The listing builds one solid part. Answer for the finished solid, in the listing's coordinates (mm). A direction names the side the tool comes from. Round coordinates to 2 decimals unless told otherwise and drop trailing zeros. Write each loop counter-clockwise with the first axis right and the second up, starting at its lowest first coordinate (ties: lowest second). Pieces come first, ordered by that corner, then holes. Notation, with made-up numbers: M -33,79 L -27,79 A21 cw -27,88 Z; hole C -21,28.5 d3. An arc over 180 degrees is marked long. One line per item, written item: value. Start each with the question number.
(1) For faces 1 (the cylindrical face through (-2.14, 9.52, 3.22)), 2 (the cylindrical face through (-17.19, 29.6, 3.22)), 3 (the cylindrical face through (-20.1, 40.8, 3.2)), determine the directions among +Z, -Z, +X, -X, +Y, -Y from which every point of the face is accessible in a straight line to the end or side of a thin tool.
(2) Consider probe 1 along Y at (x, z) = (-15.5, 4.75); probe 2 along Y at (x, z) = (-22, 2.5); probe 3 along Y at (x, z) = (-4, 4.75). Determine where each line is inside the solid, lowest interval first.
(3) Section C-C (y = 14.5) is taken. Determine the outline of the cut face in (x, z), plus the area to 3 significant figures.
(4) For a pull along Y with two mould halves and no side action, classify faces 4 (the cylindrical face through (-31.1, 39.5, 3.2)), 5 (the cylindrical face through (-24.469, 0.455, 3.219)), 6 (the cylindrical face through (-13.3, 72.9, 3.2)) as released by +Y, released by -Y, zero draft, split by the parting line, or undercut.
(5) Given P1, Ø10, axis at x = -32.5, y = 11, coming from the -Z side; P2, Ø1.9, axis at y = 22, z = 3, coming from the +X side, each flat-ended and moving along its own axis, determine where each tip first touches the part or whether it passes through.
(6) Section A-A (z = 3.5) is taken. Determine the outline of the cut face in (x, y), plus the area to 3 significant figures.
(7) Section B-B (x = -7) is taken. Determine the outline of the cut face in (y, z), plus the area to 3 significant figures.
(8) Section D-D (x = -16.5) is taken. Determine the outline of the cut face in (y, z).
```python
from build123d import *

# Parameters (mm, degrees)
F1_DEPTH = 6.35
F2_R     = 2


with BuildPart() as f1:
    # F0 (on Top) → F1 (new body)
    with BuildSketch(Plane.XY):
        Polygon((-24.87639, 0), (0, 0), (-1.76327, 10), (-17.76327, 10), (-17.76327, 30.2), (-5.325075, 30.2), (-12.9424, 73.4), (-37.289809, 73.4), (-35.52654, 63.4), (-19.52654, 63.4), (-19.52654, 40.2), (-31.964735, 40.2), align=None)
    extrude(amount=F1_DEPTH)

    # F2
    f2_edges = [f1.edges().sort_by_distance(p)[0] for p in [
        (-37.289809, 73.4, 3.175),
        (-35.52654, 63.4, 3.175),
        (-19.52654, 63.4, 3.175),
        (-31.964735, 40.2, 3.175),
        (-19.52654, 40.2, 3.175),
        (-12.9424, 73.4, 3.175),
        (-5.325075, 30.2, 3.175),
        (-17.76327, 30.2, 3.175),
        (-17.76327, 10, 3.175),
        (-1.76327, 10, 3.175),
        (0, 0, 3.175),
        (-24.87639, 0, 3.175),
    ]]
    fillet(f2_edges, radius=F2_R)


solid = f1.part
```
Recorded:
1. face 1: +Z, -Z, +X, +Y
1. face 2: +Z, -Z, +X
1. face 3: +Z, -Z, -X
2. probe 1: y = 0 to 10, 30.2 to 73.4
2. probe 2: y = 0 to 40.2, 63.4 to 73.4
2. probe 3: y = 0 to 10
3. outline: M -27.43,0 L -17.76,0 L -17.76,6.35 L -27.43,6.35 Z
3. area: 61.4 mm2
4. face 4: undercut
4. face 5: released by -Y
4. face 6: released by +Y
5. P1: passes through
5. P2: stops at x = -17.76
6. outline: M -36.88,71.05 L -35.82,65.05 A2 ccw -33.85,63.4 L -21.53,63.4 A2 cw -19.53,61.4 L -19.53,42.2 A2 cw -21.53,40.2 L -29.58,40.2 A2 ccw -31.55,37.85 L -25.17,1.65 A2 ccw -23.2,0 L -2.38,0 A2 ccw -0.41,2.35 L -1.47,8.35 A2 ccw -3.44,10 L -15.76,10 A2 cw -17.76,12 L -17.76,28.2 A2 cw -15.76,30.2 L -7.71,30.2 A2 ccw -5.74,32.55 L -12.65,71.75 A2 ccw -14.62,73.4 L -34.91,73.4 A2 ccw Z
6. area: 1,190 mm2
7. outline: M 0,0 L 10,0 L 10,6.35 L 0,6.35 Z; M 30.33,0 L 39.7,0 L 39.7,6.35 L 30.33,6.35 Z
7. area: 123 mm2
8. outline: M 0,0 L 10.14,0 L 10.14,6.35 L 0,6.35 Z; M 30.06,0 L 73.4,0 L 73.4,6.35 L 30.06,6.35 Z
